CAD build for the part. Positions are in the model's coordinates, mm. Face numbers are marked on the shaded views. A direction names the side the tool comes from. Give positions to 0.01 mm unless a question says otherwise; leave off trailing zeros. Order: outer loops, then holes, each group sorted by start corner. A loop starts at its lowest first (then second) coordinate and runs counter-clockwise, first axis right, second up. Notation, with made-up numbers: (-1.5, -39) -> (39.5, -39) arc R22 cw to (39.5, -23) -> close; hole circle Ø1 at (43.25, 12). An arc over 180 degrees is marked (long way). Answer as CSV lines item,"result".
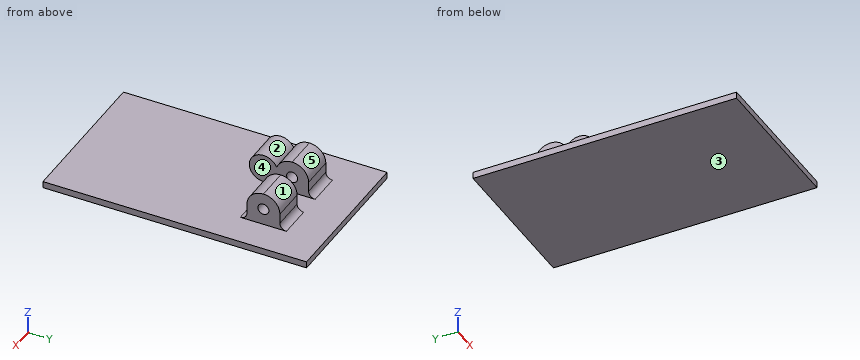
```python
from build123d import *

# Parameters (mm, degrees)
F0_W     = 15
F0_H     = 15
F1_DEPTH = 70
F2_D     = 5
F4_R     = 7.49999
F3_W     = 15
F3_H     = 15
F3_W_2   = 10
F5_DEPTH = 15
F6_R     = 3
F8_DEPTH = 15


# Not quite as in the source:
# - a fillet or chamfer is up to 0.001 mm smaller than in the source, because OpenCascade refuses the exact size


with BuildPart() as f1:
    # F0 (on Right) → F1 (new body)
    with BuildSketch(Plane.YZ):
        with Locations((92.5, 7.5)):
            Rectangle(F0_W, F0_H)
        Polygon((85, 0), (0, 0), (0, -3), (120, -3), (120, 0), (100, 0), align=None)
    extrude(amount=F1_DEPTH)

    # F2 (through all)
    with Locations(Plane(origin=(0, 0, 0), x_dir=(0, 1, 0), z_dir=(-1, 0, 0))):
        with Locations((92.5, -7.5)):
            Hole(F2_D / 2)

    # F4 (radius 7.5 in the source; OpenCascade refuses exactly that, so slightly less here)
    f4_edges = [f1.edges().sort_by_distance(p)[0] for p in [
        (35, 85, 15),
        (35, 100, 15),
    ]]
    fillet(f4_edges, radius=F4_R)

    # F3 (on face) → F5 (cut, through all)
    with BuildSketch(Plane(origin=(0, 100, 0), x_dir=(-1, 0, 0), z_dir=(0, 1, 0))):
        with Locations((-62.5, 7.5)):
            Rectangle(F3_W, F3_H)
        with Locations((-7.5, 7.5)):
            Rectangle(F3_W, F3_H)
        with Locations((-35, 7.5)):
            Rectangle(F3_W_2, F3_H)
    extrude(amount=-F5_DEPTH, mode=Mode.SUBTRACT)

    # F6
    f6_edges = [f1.edges().sort_by_distance(p)[0] for p in [
        (47.5, 85, 0),
        (22.5, 85, 0),
        (22.5, 100, 0),
        (47.5, 100, 0),
    ]]
    fillet(f6_edges, radius=F6_R)

    # F7 (on face) → F8 (join, through all)
    with BuildSketch(Plane.YZ.offset(30)):
        with BuildLine():
            ThreePointArc((85, 7.50001), (85.1162856981, 8.815593818), (85.461536824, 10.0903819596))
            ThreePointArc((85.461536824, 10.0903819596), (73.0188041666, 7.994065349), (85, 4.0358983849))
            Line((85, 4.0358983849), (85, 7.50001))
        make_face()
        with BuildLine():
            ThreePointArc((85, 4.0358983849), (85.7449979984, 5.6972243623), (86, 7.5))
            ThreePointArc((86, 7.5), (85.8639606125, 8.8228776671), (85.461536824, 10.0903819596))
            ThreePointArc((85.461536824, 10.0903819596), (85.1162856981, 8.815593818), (85, 7.50001))
            Line((85, 7.50001), (85, 4.0358983849))
        make_face()
    extrude(amount=-F8_DEPTH)


solid = f1.part
```
1) Which spindle directions (+Z, -Z, +X, -X, +Y, -Y) get a long thin tool onto all of the face, cutting with end or side? Do the marked faces 4 and 5. Say none if no direction does.
Data:
face 4,"+Z, +Y, -Y"
face 5,"+Z, +X, -X, +Y"
2) Band-saw the part on A-A, the plane y = 79.5. Write the cut outline in (x, z).
Data:
outline,"(0, -3) -> (70, -3) -> (70, 0) -> (0, 0) -> close; (15, 1) -> (30, 1) -> (30, 14) -> (15, 14) -> close"
3) Pin check, flat tips, straight feed: P1, Ø5, axis at x = 31.5, z = 12, coming from the -Y side; P2, Ø7.5, axis at y = 88.5, z = 7, coming from the -X side; P3, Ø2.5, axis at x = 47, z = 5.5, coming from the +Y side. Stop position of each tip, or through.
Data:
P1,"stops at y = 73.5"
P2,"stops at x = 15"
P3,"stops at y = 100"
4) Pull direction Z, two halves, no side cores. Call the marked faces 1, 2 and 3: pulls with the +Z half, pulls with the -Z half, needs draft (parallel to the pull), parting line crosses it, or undercut.
Data:
face 1,"pulls with the +Z half"
face 2,"undercut"
face 3,"pulls with the -Z half"
5) Wall check: line 1 along X through (y, z) = (96, 4); line 2 along Z through (x, y) = (43.75, 92.5); line 3 along X through (y, z) = (84, 12). Give the ranges that are in metal, low to high. Write a range as [from, to].
Data:
line 1,"x = [15, 30], [40, 55]"
line 2,"z = [-3, 5], [10, 15]"
line 3,"x = [15, 30]"
6) Band-saw the part on D-D, the plane y = 16.5. Write the cut outline in (x, z), then the cut area to 3 significant figures.
Data:
outline,"(0, -3) -> (70, -3) -> (70, 0) -> (0, 0) -> close"
area,"210 mm2"
